```python
from build123d import *
from OCP.BRepFilletAPI import BRepFilletAPI_MakeChamfer

# Parameters (mm, degrees)
SKETCH1_W           = 213
SKETCH1_H           = 71
BOSS_EXTRUDE1_DEPTH = 34
CHAMFER1_SIZE       = 1
CHAMFER1_SIZE2      = 0.176326981
CHAMFER2_SIZE       = 1
CHAMFER2_SIZE2      = 0.176326981
SKETCH3_W           = 23.647346038
SKETCH3_H           = 16.197572193
SKETCH3_W_2         = 4
SKETCH3_H_2         = 13.380603116
SKETCH3_H_3         = 13.392122804
SKETCH3_H_4         = 13.411553204
SKETCH3_H_5         = 13.439263392
CUT_EXTRUDE2_DEPTH  = 1
SKETCH4_W           = 6
SKETCH4_H           = 1
CUT_EXTRUDE3_DEPTH  = 1


with BuildPart() as part:
    # Sketch1 → Boss-Extrude1 (new body)
    with BuildSketch(Plane.XY):
        with Locations((61.169898141, -8.554853616)):
            Rectangle(SKETCH1_W, SKETCH1_H)
    extrude(amount=BOSS_EXTRUDE1_DEPTH)

    # Chamfer1: one chamfer whose edges measure the first distance from different faces: ONE call of the kernel's chamfer builder (chamfer() names one face for all edges)
    chamfer1_edges_1 = [part.edges().sort_by_distance(p)[0] for p in [
        (-45.330101859, -8.554853616, 34),
    ]]
    chamfer1_side_1 = [part.faces().sort_by_distance(p)[0] for p in [
        (61.169898141, -8.554853616, 34),
    ]]
    chamfer1_edges_2 = [part.edges().sort_by_distance(p)[0] for p in [
        (-45.330101859, -8.554853616, 0),
    ]]
    chamfer1_side_2 = [part.faces().sort_by_distance(p)[0] for p in [
        (61.169898141, -8.554853616, 0),
    ]]
    chamfer1_edges_3 = [part.edges().sort_by_distance(p)[0] for p in [
        (-45.330101859, 26.945146384, 17),
    ]]
    chamfer1_side_3 = [part.faces().sort_by_distance(p)[0] for p in [
        (61.169898141, 26.945146384, 17),
    ]]
    chamfer1 = BRepFilletAPI_MakeChamfer(part.part.solid().wrapped)
    for e in chamfer1_edges_1:
        chamfer1.Add(CHAMFER1_SIZE, CHAMFER1_SIZE2, e.wrapped, chamfer1_side_1[0].wrapped)  # the first distance lies on this face
    for e in chamfer1_edges_2:
        chamfer1.Add(CHAMFER1_SIZE, CHAMFER1_SIZE2, e.wrapped, chamfer1_side_2[0].wrapped)  # the first distance lies on this face
    for e in chamfer1_edges_3:
        chamfer1.Add(CHAMFER1_SIZE, CHAMFER1_SIZE2, e.wrapped, chamfer1_side_3[0].wrapped)  # the first distance lies on this face
    add(Compound.cast(chamfer1.Shape()), mode=Mode.REPLACE)

    # Chamfer2: one chamfer whose edges measure the first distance from different faces: ONE call of the kernel's chamfer builder (chamfer() names one face for all edges)
    chamfer2_edges_1 = [part.edges().sort_by_distance(p)[0] for p in [
        (167.669898141, -8.554853616, 34),
    ]]
    chamfer2_side_1 = [part.faces().sort_by_distance(p)[0] for p in [
        (61.669898141, -8.554853616, 34),
    ]]
    chamfer2_edges_2 = [part.edges().sort_by_distance(p)[0] for p in [
        (167.669898141, -8.554853616, 0),
    ]]
    chamfer2_side_2 = [part.faces().sort_by_distance(p)[0] for p in [
        (61.669898141, -8.554853616, 0),
    ]]
    chamfer2_edges_3 = [part.edges().sort_by_distance(p)[0] for p in [
        (167.669898141, 26.945146384, 17),
    ]]
    chamfer2_side_3 = [part.faces().sort_by_distance(p)[0] for p in [
        (61.669898141, 26.945146384, 17),
    ]]
    chamfer2 = BRepFilletAPI_MakeChamfer(part.part.solid().wrapped)
    for e in chamfer2_edges_1:
        chamfer2.Add(CHAMFER2_SIZE, CHAMFER2_SIZE2, e.wrapped, chamfer2_side_1[0].wrapped)  # the first distance lies on this face
    for e in chamfer2_edges_2:
        chamfer2.Add(CHAMFER2_SIZE, CHAMFER2_SIZE2, e.wrapped, chamfer2_side_2[0].wrapped)  # the first distance lies on this face
    for e in chamfer2_edges_3:
        chamfer2.Add(CHAMFER2_SIZE, CHAMFER2_SIZE2, e.wrapped, chamfer2_side_3[0].wrapped)  # the first distance lies on this face
    add(Compound.cast(chamfer2.Shape()), mode=Mode.REPLACE)

    # Sketch3 → Cut-Extrude2 (cut)
    with BuildSketch(Plane.ZY.offset(45.330101859)):
        with Locations((17, -25.758486194)):
            Rectangle(SKETCH3_W, SKETCH3_H)
        with Locations((8.705796188, -25.859092232)):
            Rectangle(SKETCH3_W_2, SKETCH3_H_2, mode=Mode.SUBTRACT)
        with Locations((14.235265396, -25.864852076)):
            Rectangle(SKETCH3_W_2, SKETCH3_H_3, mode=Mode.SUBTRACT)
        with Locations((19.764734604, -25.874567276)):
            Rectangle(SKETCH3_W_2, SKETCH3_H_4, mode=Mode.SUBTRACT)
        with Locations((25.294203812, -25.88842237)):
            Rectangle(SKETCH3_W_2, SKETCH3_H_5, mode=Mode.SUBTRACT)
    extrude(amount=-CUT_EXTRUDE2_DEPTH, mode=Mode.SUBTRACT)

    # Sketch4 → Cut-Extrude3 (cut)
    with BuildSketch(Plane.ZY.offset(45.330101859)):
        Polygon((8.176326981, -35.85727229), (9.176326981, -35.85727229), (9.176326981, -38.35727229), (11.676326981, -38.35727229), (11.676326981, -39.35727229), (9.176326981, -39.35727229), (9.176326981, -41.85727229), (8.176326981, -41.85727229), (8.176326981, -39.35727229), (5.676326981, -39.35727229), (5.676326981, -38.35727229), (8.176326981, -38.35727229), align=None)
        with Locations((25.720428724, -38.85727229)):
            Rectangle(SKETCH4_W, SKETCH4_H)
    extrude(amount=-CUT_EXTRUDE3_DEPTH, mode=Mode.SUBTRACT)


solid = part.part
```
Input: part model. Units: mm. Frame: model coordinates. Round coordinates to 2 decimals unless told otherwise and drop trailing zeros. Answer in a Markdown table with one row per item. Add a question column.
1. Mould query, pull axis Z, two halves, no side actions, for faces 1 (the face through (-44.33, -26, 17)), 2 (the face through (60, -8, 0)), 3 (the face through (-44.33, -39, 9)), 4 (the face through (-45.33, -26, 25)). Classes: released by +Z, released by -Z, zero draft, split by the parting line, or undercut.
2. Contact query for flat-ended pins moving along their axis: pin 1 (1.1 mm diameter, centred on x = -45, z = 24.5, fed in from +Y); pin 2 (1.8 mm diameter, centred on y = -39, z = 10, fed in from -X); pin 3 (0.5 mm diameter, centred on x = -45, y = -23.5, fed in from -Z); pin 4 (0.8 mm diameter, centred on x = -45, y = -28, fed in from +Z). Output: stop coordinate, or through.
3. Ray query, probe 1 along X at (y, z) = (-38.5, 10.5). Return the intervals inside material, ascending.
Values follow:
| question | item | result |
|---|---|---|
| 1 | face 1 | undercut |
| 1 | face 2 | released by -Z |
| 1 | face 3 | undercut |
| 1 | face 4 | zero draft |
| 2 | pin 1 | y = 26.92 |
| 2 | pin 2 | x = -45.33 |
| 2 | pin 3 | z = 0.07 |
| 2 | pin 4 | z = 33.95 |
| 3 | probe 1 | -44.33 to 167.67 |
